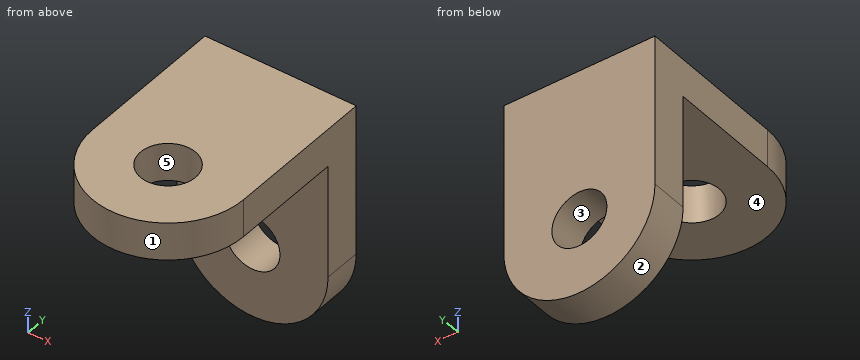
from build123d import *

# Parameters (mm, degrees)
F0_R     = 2.3114
F1_DEPTH = 3.175
F2_R     = 2.3114
F3_DEPTH = 3.175


with BuildPart() as f1:
    # F0 (on Top) → F1 (new body)
    with BuildSketch(Plane.XY):
        with BuildLine():
            Line((-6.35, 12.7), (-6.35, 0))
            ThreePointArc((-6.35, 0), (0, -6.35), (6.35, 0))
            Line((6.35, 0), (6.35, 12.7))
            Line((6.35, 12.7), (-6.35, 12.7))
        make_face()
        Circle(F0_R, mode=Mode.SUBTRACT)
    extrude(amount=F1_DEPTH)

    # F2 (on face) → F3 (join)
    with BuildSketch(Plane(origin=(0, 12.7, 0), x_dir=(-1, 0, 0), z_dir=(0, 1, 0))):
        with BuildLine():
            Line((-6.35, 3.175), (-6.35, -9.525))
            ThreePointArc((-6.35, -9.525), (0, -15.875), (6.35, -9.525))
            Line((6.35, -9.525), (6.35, 3.175))
            Line((6.35, 3.175), (-6.35, 3.175))
        make_face()
        with Locations((0, -9.525)):
            Circle(F2_R, mode=Mode.SUBTRACT)
    extrude(amount=-F3_DEPTH)


solid = f1.part
Design review of the part built by this model. Coordinates are the model's own, in mm. Face numbers are marked on the shaded views. A direction names the side the tool comes from. Give positions to 0.01 mm unless a question says otherwise; leave off trailing zeros. Order: outer loops, then holes, each group sorted by start corner. A loop starts at its lowest first (then second) coordinate and runs counter-clockwise, first axis right, second up. Notation, with made-up numbers: (88.25, 69) - (141.25, 69) arc R29 ccw to (141.25, 89) - close; hole circle Ø4 at (-12.5, 19.25). An arc over 180 degrees is marked (long way). Use CSV: the item, a comma, the result in double quotes. Start each with the question number.
Q1. Draft analysis for pull direction Z (two halves, no side actions). For the marked faces 1, 2 and 3, state which applies: pulls with the +Z half, pulls with the -Z half, needs draft (parallel to the pull), parting line crosses it, or undercut.
Q2. Take a section at A-A (x = 0). State the section outline as (y, z) points (3 decimals), and give its area (3 significant figures).
Q3. For P1, Ø7.5, axis at x = 0, y = 0, coming from the -Z side; P2, Ø6, axis at x = 4, z = -10, coming from the -Y side (3 decimals), all flat-tipped, find the tip position at first contact; note any pin that passes through.
Q4. For line 1 (Y direction, x = 0, z = 1.8); line 2 (Z direction, x = 0, y = 10.2) (3 decimals); line 3 (Z direction, x = 1, y = -2.5) (3 decimals), list the stretches that pass through material, from the lowest coordinate up.
Q5. Take a section at C-C (z = -11.5). State the section outline as (x, y) points (3 decimals).
Q6. Take a section at B-B (z = 1.5). State the section outline as (x, y) points.
Q7. Take a section at D-D (y = 4.75). State the section outline as (x, z) points (3 decimals).
Q8. Machinability: for the marked faces 4 and 5, which of the approach directions +Z, -Z, +X, -X, +Y, -Y give a long, thin tool a straight path to every point of the face, cutting with its end or side? Answer none if there is none.
Calculated:
1,face 1,"needs draft"
1,face 2,"pulls with the -Z half"
1,face 3,"undercut"
2,outline,"(-6.35, 0) - (-2.311, 0) - (-2.311, 3.175) - (-6.35, 3.175) - close; (2.311, 0) - (9.525, 0) - (9.525, -7.214) - (12.7, -7.214) - (12.7, 3.175) - (2.311, 3.175) - close; (9.525, -15.875) - (12.7, -15.875) - (12.7, -11.836) - (9.525, -11.836) - close"
2,area,"81.5 mm²"
3,P1,"stops at z = 0"
3,P2,"stops at y = 9.525"
4,line 1,"y = -6.35 to -2.31, 2.31 to 12.7"
4,line 2,"z = -15.875 to -11.836, -7.214 to 3.175"
4,line 3,"z = 0 to 3.175"
5,outline,"(-6.035, 9.525) - (-1.201, 9.525) - (-1.201, 12.7) - (-6.035, 12.7) - close; (1.201, 9.525) - (6.035, 9.525) - (6.035, 12.7) - (1.201, 12.7) - close"
6,outline,"(-6.35, 0) arc R6.35 ccw to (6.35, 0) - (6.35, 12.7) - (-6.35, 12.7) - close; hole circle Ø4.62 at (0, 0)"
7,outline,"(-6.35, 0) - (6.35, 0) - (6.35, 3.175) - (-6.35, 3.175) - close"
8,face 4,"-Z, +X, -X, -Y"
8,face 5,"+Z, -Z"
